from build123d import *

# Parameters (mm, degrees)
BOSS_EXTRUDE1_DEPTH = 5


with BuildPart() as part:
    # Sketch1 → Boss-Extrude1 (new body)
    with BuildSketch(Plane(origin=(0, 0, 0), x_dir=(1, 0, 0), z_dir=(0, 1, 0))):
        with BuildLine():
            Line((15, 40), (0, 40))
            Line((0, 40), (0, 14.1))
            ThreePointArc((0, 14.1), (2.899137803, 12.899137803), (4.1, 10))
            ThreePointArc((4.1, 10), (2.899137803, 7.100862197), (0, 5.9))
            Line((0, 5.9), (0, 0))
            Line((0, 0), (15, 0))
            Line((15, 0), (15, 40))
        make_face()
        with BuildLine():
            Line((0, 65.9), (0, 40))
            Line((0, 40), (15, 40))
            Line((15, 40), (15, 80))
            Line((15, 80), (0, 80))
            Line((0, 80), (0, 74.1))
            ThreePointArc((0, 74.1), (2.899137803, 72.899137803), (4.1, 70))
            ThreePointArc((4.1, 70), (2.899137803, 67.100862197), (0, 65.9))
        make_face()
    extrude(amount=BOSS_EXTRUDE1_DEPTH)


solid = part.part
The model under review builds one solid part; all positions refer to its coordinate system, in mm. Give positions to 0.01 mm unless a question says otherwise; leave off trailing zeros. Loops run counter-clockwise (first coordinate to the right, second up) from the corner with the lowest first, then second, coordinate; pieces in that order, holes last. Notation, with made-up numbers: (33.25, 47) -> (40.25, 47) arc R36 ccw to (40.25, 82) -> close; hole circle Ø9 at (21.25, 68). An arc over 180 degrees is marked (long way). Put each result on its own line as item: value. Start each with the question number.
1. We need section A-A on y = 1.2. State the section outline as (x, z) points, then the cut area to 3 significant figures.
2. Clearance check with a flat-ended pin moving along its axis: P1, Ø8, axis at x = 6.5, z = -12, coming from the -Y side. State where the tip first meets the part, or that it passes through.
3. Wall thickness on probe 1 along Z at (x, y) = (2, 4.4); probe 2 along X at (y, z) = (4.35, -9): over which ranges is each line inside the solid? List them lowest first.
Determined:
1. outline: (0, -80) -> (15, -80) -> (15, 0) -> (0, 0) -> (0, -5.9) arc R4.1 cw to (0, -14.1) -> (0, -65.9) arc R4.1 cw to (0, -74.1) -> close
1. area: 1,150 mm^2
2. P1: y = 0
3. probe 1: -80 to -73.58, -66.42 to -13.58, -6.42 to 0
3. probe 2: 3.98 to 15
